Study the drawing (mm; zero at the part's minimum x, y, z) and answer. A direction names the side the tool comes from. Round coordinates to 2 decimals unless told otherwise and drop trailing zeros. Write each loop counter-clockwise with the first axis right and the second up, starting at its lowest first coordinate (ties: lowest second). Pieces come first, ordered by that corner, then holes. Notation, with made-up numbers: (84.5, 51) - (128.5, 51) arc R18 ccw to (128.5, 68) - close; hole circle Ø10 at (67.25, -11). An arc over 180 degrees is marked (long way). Return JSON: item names as keys, results as strings. Group by question number.
(1) Which of the six approach directions +Z, -Z, +X, -X, +Y, -Y give full straight-line access (tool end or side, diameter ignored) to the marked faces 1 and 2?
(2) Section A-A, the plane y = 2 is taken. Write down the section's boundary in (x, z) (3 decimals).
(3) Section B-B, the plane x = 2 is taken. Write down the section's boundary in (y, z) (3 decimals).
(4) This flat-tipped pin is pushed along its axis until it touches: pin 1 (2 mm diameter, centred on y = 1.5, z = 1, fed in from +X). Where does it stop, or does it pass through?
(5) Section C-C, the plane z = 3 is taken. Write down the section's boundary in (x, y), then the cut area to 3 significant figures.
(6) Section D-D, the plane y = 2.9 is taken. Write down the section's boundary in (x, z) (3 decimals).
(7) Find the intervals of material crossed by line 1 along X through (y, z) = (1.95, 5.75); line 2 along Z through (x, y) = (0.7, 3.1); line 3 along X through (y, z) = (2.9, 3.5), in increasing order. Write a range as [from, to].
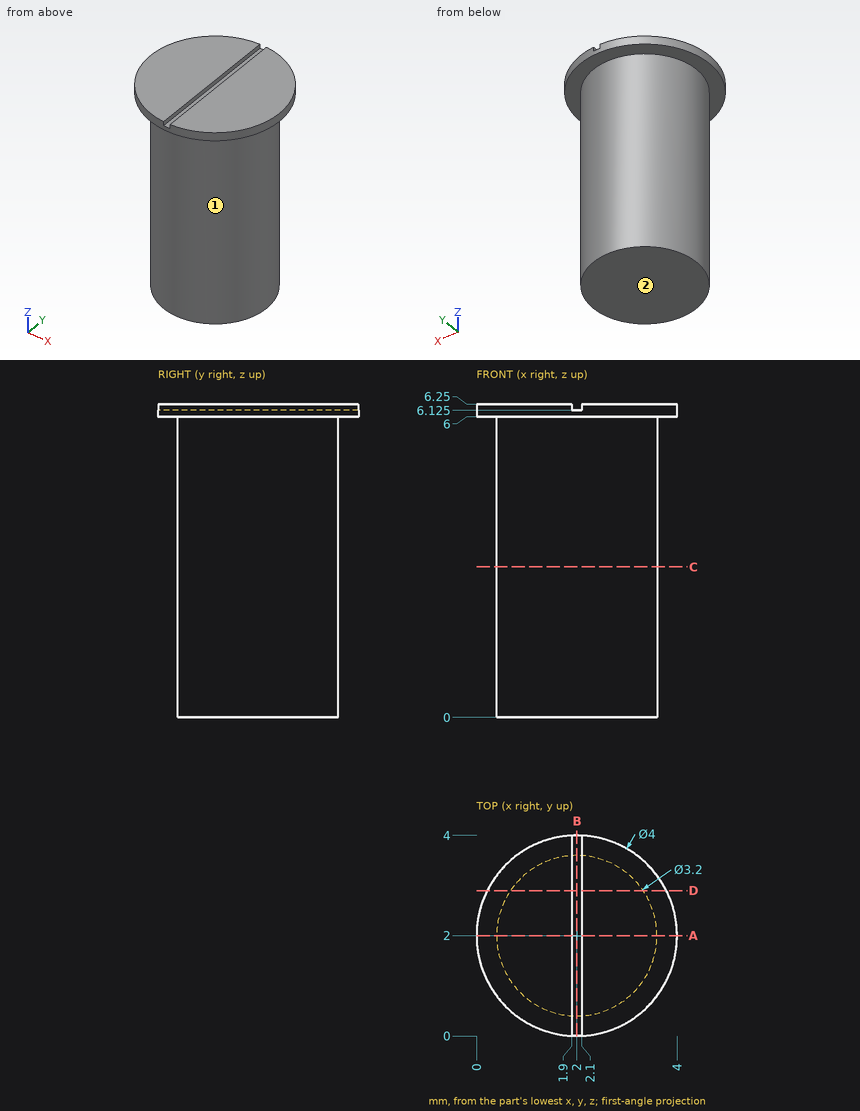
Working result:
{
 "1": {"face 1": "-Z", "face 2": "-Z, +X, -X, +Y, -Y"},
 "2": {"outline": "(0, 6) - (0.4, 6) - (0.4, 0) - (3.6, 0) - (3.6, 6) - (4, 6) - (4, 6.25) - (2.1, 6.25) - (2.1, 6.125) - (1.9, 6.125) - (1.9, 6.25) - (0, 6.25) - close"},
 "3": {"outline": "(0, 6) - (0.4, 6) - (0.4, 0) - (3.6, 0) - (3.6, 6) - (4, 6) - (4, 6.125) - (0, 6.125) - close"},
 "4": {"pin 1": "stops at x = 3.6"},
 "5": {"outline": "circle Ø3.2 at (2, 2)", "area": "8.04 mm^2"},
 "6": {"outline": "(0.214, 6) - (0.677, 6) - (0.677, 0) - (3.323, 0) - (3.323, 6) - (3.786, 6) - (3.786, 6.25) - (2.1, 6.25) - (2.1, 6.125) - (1.9, 6.125) - (1.9, 6.25) - (0.214, 6.25) - close"},
 "7": {"line 1": "x = [0.4, 3.6]", "line 2": "z = [6, 6.25]", "line 3": "x = [0.68, 3.32]"}
}
